Design review of the part built by this model. Coordinates are the model's own, in mm. A direction names the side the tool comes from. Give positions to 0.01 mm unless a question says otherwise; leave off trailing zeros. Loops run counter-clockwise (first coordinate to the right, second up) from the corner with the lowest first, then second, coordinate; pieces in that order, holes last. Notation, with made-up numbers: M 17.5,-30.75 L 32.5,-30.75 A25 cw 32.5,7.25 Z; hole C 44,14.25 d2. An arc over 180 degrees is marked long. Use CSV: the item, a comma, the result in double quotes.
from build123d import *

# Parameters (mm, degrees)
SKETCH1_R               = 2.25
BOSS_EXTRUDE1_DEPTH     = 5
CUT_EXTRUDE1_DEPTH      = 53.646794774
CUT_EXTRUDE2_DEPTH      = 53.646794774
CUT_EXTRUDE2_DEPTH_BACK = 53.646794774
SKETCH4_R               = 1.4
SKETCH4_W               = 23.4
SKETCH4_H               = 13
FILLET1_R               = 5
FILLET2_R               = 1
FILLET3_R               = 2
SKETCH5_R               = 7
CUT_EXTRUDE3_DEPTH      = 53.646794774


with BuildPart() as part:
    # Sketch1 → Boss-Extrude1 (new body)
    with BuildSketch(Plane(origin=(0, 0, 0), x_dir=(1, 0, 0), z_dir=(0, 1, 0))):
        with BuildLine():
            Line((0, 9), (15.123161628, 9))
            Line((15.123161628, 9), (24.12692112, 33.737625896))
            ThreePointArc((24.12692112, 33.737625896), (32.137625896, 37.47307888), (35.87307888, 29.462374104))
            Line((35.87307888, 29.462374104), (20.41803863, -13))
            Line((20.41803863, -13), (4.868831591, -32.31879815))
            ThreePointArc((4.868831591, -32.31879815), (2.699074986, -34.037153024), (0, -34.65))
            Line((0, -34.65), (0, -30.65))
            ThreePointArc((0, -30.65), (2.25, -28.4), (0, -26.15))
            Line((0, -26.15), (0, -9))
            Line((0, -9), (0, 9))
        make_face()
        with Locations(Location((30, 31.6, 0), (0, 0, 270))):
            Circle(SKETCH1_R, mode=Mode.SUBTRACT)
    boss_extrude1 = extrude(amount=BOSS_EXTRUDE1_DEPTH)

    # Mirror1: Boss-Extrude1 across plane
    add(boss_extrude1.mirror(Plane(origin=(0, 0, 0), x_dir=(0, 0, 1), z_dir=(1, 0, 0))))

    # Sketch3 → Cut-Extrude1 (cut, symmetric)
    with BuildSketch(Plane(origin=(0, 5, 0), x_dir=(1, 0, 0), z_dir=(0, 1, 0))):
        Polygon((-15.123161628, 9), (-24.12692112, 33.737625896), (-24.12692112, 20.448726138), (-19.05, 6.5), (0, 6.5), (0, 9), align=None)
    cut_extrude1 = extrude(amount=CUT_EXTRUDE1_DEPTH, both=True, mode=Mode.SUBTRACT)

    # Mirror2: Cut-Extrude1 across plane
    add(cut_extrude1.mirror(Plane(origin=(0, 0, 0), x_dir=(0, 0, 1), z_dir=(1, 0, 0))), mode=Mode.SUBTRACT)

    # Sketch4 → Cut-Extrude2 (cut, two sides: drawn at the far end of the back side and taken through both)
    with BuildSketch(Plane(origin=(0, 5, 0), x_dir=(1, 0, 0), z_dir=(0, 1, 0)).offset(-CUT_EXTRUDE2_DEPTH_BACK)):
        with Locations(Location((6.5, 0, 0), (0, 0, 270))):
            Circle(SKETCH4_R)
        with Locations(Location((-21.2, 0, 0), (0, 0, 270))):
            Circle(SKETCH4_R)
        with Locations((-7.35, 0)):
            Rectangle(SKETCH4_W, SKETCH4_H)
    extrude(amount=CUT_EXTRUDE2_DEPTH + CUT_EXTRUDE2_DEPTH_BACK, mode=Mode.SUBTRACT)

    # Fillet1
    fillet1_edges = [part.edges().sort_by_distance(p)[0] for p in [
        (20.41803863, 2.5, 13),
        (-20.41803863, 2.5, 13),
        (-24.12692112, 2.5, -20.448726138),
        (19.05, 2.5, -6.5),
        (24.12692112, 2.5, -20.448726138),
    ]]
    fillet(fillet1_edges, radius=FILLET1_R)

    # Fillet2
    fillet2_edges = [part.edges().sort_by_distance(p)[0] for p in [
        (4.35, 2.5, 6.5),
        (-19.05, 2.5, 6.5),
    ]]
    fillet(fillet2_edges, radius=FILLET2_R)

    # Fillet3
    fillet3_edges = [part.edges().sort_by_distance(p)[0] for p in [
        (4.35, 2.5, -6.5),
    ]]
    fillet(fillet3_edges, radius=FILLET3_R)

    # Sketch5 → Cut-Extrude3 (cut, through all)
    with BuildSketch(Plane(origin=(0, 5, 0), x_dir=(1, 0, 0), z_dir=(0, 1, 0))):
        with Locations(Location((0, -16, 0), (0, 0, 270))):
            Circle(SKETCH5_R)
    extrude(amount=-CUT_EXTRUDE3_DEPTH, mode=Mode.SUBTRACT)


solid = part.part
(1) Machinability: for faces 1 (the flat face through (4.35, 2, 1)), 2 (the cylindrical face through (-22.567, 2.465, -0.303)), which of the approach directions +Z, -Z, +X, -X, +Y, -Y give a long, thin tool a straight path to every point of the face, cutting with its end or side? Answer none if there is none.
A:
face 1,"-Z, +Y, -Y"
face 2,"+Y, -Y"
(2) We need section C-C on y = 1.9. Count the separate pieces of the cut face and the enclosed holes in it, then the cut area to 3 significant figures.
A:
separate pieces,"1"
enclosed holes,"6"
area,"1,510 mm²"
(3) The part is to be moulded in two halves that separate along X. For faces 3 (the flat face through (5, 0, -4)), 4 (the flat face through (-28.394, 2.465, -8.913)), 5 (the flat face through (-24.127, 3, -28)), 6 (the cylindrical face through (-30.676, 2.465, -29.454)), say which applies: released by +X, released by -X, zero draft, split by the parting line, or undercut.
A:
face 3,"zero draft"
face 4,"released by -X"
face 5,"undercut"
face 6,"undercut"
(4) We need section D-D on z = 0. State the section outline as (x, y) points, then the cut area to 3 significant figures.
A:
outline,"M -25.15,0 L -22.6,0 L -22.6,5 L -25.15,5 Z; M -19.8,0 L -19.05,0 L -19.05,5 L -19.8,5 Z; M 4.35,0 L 5.1,0 L 5.1,5 L 4.35,5 Z; M 7.9,0 L 25.15,0 L 25.15,5 L 7.9,5 Z"
area,"106 mm²"
(5) Wall thickness on line 1 along X through (y, z) = (3.2, -31.6); line 2 along X through (y, z) = (3.45, 0); line 3 along Z through (x, y) = (6, 2.15): over which ranges is each line inside the solid? List them lowest first. Write a range as [from, to].
A:
line 1,"[-36.25, -32.25], [-27.75, -24.13], [24.13, 27.75], [32.25, 36.25]"
line 2,"[-25.15, -22.6], [-19.8, -19.05], [4.35, 5.1], [7.9, 25.15]"
line 3,"[-6.47, -1.31], [1.31, 12.39], [19.61, 30.91]"
(6) We need section B-B on z = 28.4. State the section outline as (x, y) points, then the cut area to 3 significant figures.
A:
outline,"M -8.02,0 L -2.25,0 L -2.25,5 L -8.02,5 Z; M 2.25,0 L 8.02,0 L 8.02,5 L 2.25,5 Z"
area,"57.7 mm²"
(7) We need section A-A on x = 29. State the section outline as (y, z) points.
A:
outline,"M 0,-37.77 L 5,-37.77 L 5,-33.62 L 0,-33.62 Z; M 0,-29.58 L 5,-29.58 L 5,-10.58 L 0,-10.58 Z"
(8) Clearance check with flat-ended pins moving along their axes: P1, Ø3.5, axis at x = 30, z = -31.6, coming from the +Y side; P2, Ø2.5, axis at y = 2, z = -25.5, coming from the +X side; P3, Ø2.5, axis at y = 2, z = -1, coming from the -X side; P4, Ø2.5, axis at x = 9, y = 3.5, coming from the -Z side. State where each tip first meets the part, or that it passes through.
A:
P1,"through"
P2,"x = 34.89"
P3,"x = -25.97"
P4,"z = -6.5"
